Can you work these out from the model? Positions are in its coordinate system, mm. A direction names the side the tool comes from. Round coordinates to 2 decimals unless told otherwise and drop trailing zeros. Write each loop counter-clockwise with the first axis right and the second up, starting at its lowest first coordinate (ties: lowest second). Pieces come first, ordered by that corner, then holes. Notation, with made-up numbers: M 29,88 L 46,88 A9 ccw 46,103 Z; hole C 40,5.5 d7. An arc over 180 degrees is marked long. Answer as a JSON object with one key per item and string values. Group by question number.
1) Suppose I cut it at D-D, the plane y = -10. State how many separate pieces and enclosed holes the cut face has, and give its area (3 significant figures).
2) Suppose I cut it at B-B, the plane x = -49. Write out the boundary of the cut face in (y, z).
3) If we mould it in two halves opening along Y, with no side actions, what happens to faces 1 (the cylindrical face through (40.986, -6.025, 37.846)), 2 (the flat face through (41, -30.277, 49)), 3 (the flat face through (17, -4, 63))? For each: +Y half, -Y half, draft (parallel to the pull), parting line (faces both ways), or undercut.
4) On a 3-axis mill with a long thin cutter (end or side, diameter ignored), from which of +Z, -Z, +X, -X, +Y, -Y can I reach the whole of each face in a straight line? I mean faces 4 (the flat face through (-91, 2.723, 69)), 5 (the flat face through (-31, 6.873, 115)), 6 (the flat face through (-31, 5, 100)), 7 (the cylindrical face through (-39.773, -26.25, 0.74)). Say none if no direction works.
5) Please list where these lines run through material, in increasing order: L1, parallel to X at y = -25.5, z = 65; L2, parallel to X at y = -9, z = 114.5; L3, parallel to Y at x = -44, z = 41. Write a range as [from, to].
6) I'm going to push flat-ended pins straight in: pin 1 Ø12 at (x, z) = (0.5, 113.5) entering from -Y; pin 2 Ø1 at (x, z) = (-55, 109.5) entering from -Y; pin 3 Ø10 at (y, z) = (-8.5, 114.5) entering from -X. Where does each tip first touch, or does it pass through?
7) Suppose I cut it at C-C, the plane z = 45. Write out the boundary of the cut face in (x, y), and give its area (3 significant figures).
8) Suppose I cut it at A-A, the plane z = 106.5. Write out the boundary of the cut face in (x, y).
from build123d import *

# Parameters (mm, degrees)
BOSS_EXTRUDE2_DEPTH = 100
BOSS_EXTRUDE3_DEPTH = 30
SKETCH10_R          = 7.5
CUT_EXTRUDE2_DEPTH  = 210
SKETCH15_R          = 1.5
CUT_EXTRUDE3_DEPTH  = 10
SKETCH16_W          = 24
SKETCH16_H          = 12
BOSS_EXTRUDE5_DEPTH = 2
SKETCH17_W          = 3
SKETCH17_H          = 12
BOSS_EXTRUDE6_DEPTH = 25
SKETCH19_R          = 3.5
CUT_EXTRUDE4_DEPTH  = 1
SKETCH20_R          = 1.55
CUT_EXTRUDE5_DEPTH  = 3
SKETCH21_W          = 45
SKETCH21_H          = 1.5
BOSS_EXTRUDE7_DEPTH = 35
SKETCH23_R          = 8.25
CUT_EXTRUDE6_DEPTH  = 40
CUT_EXTRUDE7_DEPTH  = 40


with BuildPart() as part:
    # Sketch3 → Boss-Extrude2 (new body)
    with BuildSketch(Plane.XY):
        Polygon((-106.54853621, -30.277349769), (-106.54853621, 11.722650231), (43.45146379, 11.722650231), (43.45146379, -30.277349769), (38.45146379, -30.277349769), (38.45146379, 4.722650231), (-101.54853621, 4.722650231), (-101.54853621, -30.277349769), align=None)
    extrude(amount=BOSS_EXTRUDE2_DEPTH)

    # Sketch4 → Boss-Extrude3 (add)
    with BuildSketch(Plane.XY.offset(100)):
        with BuildLine():
            Line((-102.69853621, -0.277349769), (-102.69853621, -20.277349769))
            ThreePointArc((-102.69853621, -20.277349769), (-104.04853621, -21.627349769), (-105.39853621, -20.277349769))
            Line((-105.39853621, -20.277349769), (-105.39853621, -0.277349769))
            ThreePointArc((-105.39853621, -0.277349769), (-104.04853621, 1.072650231), (-102.69853621, -0.277349769))
        make_face()
        with BuildLine():
            Line((-56.54853621, 9.572650231), (-6.54853621, 9.572650231))
            ThreePointArc((-6.54853621, 9.572650231), (-5.19853621, 8.222650231), (-6.54853621, 6.872650231))
            Line((-6.54853621, 6.872650231), (-56.54853621, 6.872650231))
            ThreePointArc((-56.54853621, 6.872650231), (-57.89853621, 8.222650231), (-56.54853621, 9.572650231))
        make_face()
        with BuildLine():
            Line((42.45146379, -0.277349769), (42.45146379, -20.277349769))
            ThreePointArc((42.45146379, -20.277349769), (40.95146379, -21.777349769), (39.45146379, -20.277349769))
            Line((39.45146379, -20.277349769), (39.45146379, -0.277349769))
            ThreePointArc((39.45146379, -0.277349769), (40.95146379, 1.222650231), (42.45146379, -0.277349769))
        make_face()
    extrude(amount=BOSS_EXTRUDE3_DEPTH)

    # Sketch10 → Cut-Extrude2 (cut)
    with BuildSketch(Plane(origin=(43.45146379, 0, 0), x_dir=(0, 0, -1), z_dir=(1, 0, 0))):
        with Locations((-45, -8.277349769)):
            Circle(SKETCH10_R)
    extrude(amount=-CUT_EXTRUDE2_DEPTH, mode=Mode.SUBTRACT)

    # Sketch15 → Cut-Extrude3 (cut)
    with BuildSketch(Plane(origin=(0, 11.722650231, 0), x_dir=(1, 0, 0), z_dir=(0, 1, 0))):
        with Locations(Location((-31.54853621, -4.714245873, 0), (0, 0, 270))):
            Circle(SKETCH15_R)
    extrude(amount=-CUT_EXTRUDE3_DEPTH, mode=Mode.SUBTRACT)

    # Sketch16 → Boss-Extrude5 (add)
    with BuildSketch(Plane.XZ.offset(-4.722650231)):
        with Locations((26.45146379, 69)):
            Rectangle(SKETCH16_W, SKETCH16_H)
    boss_extrude5 = extrude(amount=BOSS_EXTRUDE5_DEPTH)

    # Sketch17 → Boss-Extrude6 (add)
    with BuildSketch(Plane(origin=(0, 2.722650231, 0), x_dir=(-1, 0, 0), z_dir=(0, -1, 0))):
        with Locations((-15.95146379, -69)):
            Rectangle(SKETCH17_W, SKETCH17_H)
    boss_extrude6 = extrude(amount=BOSS_EXTRUDE6_DEPTH)

    # Sketch19 → Cut-Extrude4 (cut)
    with BuildSketch(Plane.ZY.offset(-14.45146379)):
        with Locations((69.485133357, 0.222650231)):
            Circle(SKETCH19_R)
        with Locations((69.485133357, -17.777349769)):
            Circle(SKETCH19_R)
    cut_extrude4 = extrude(amount=-CUT_EXTRUDE4_DEPTH, mode=Mode.SUBTRACT)

    # Sketch20 → Cut-Extrude5 (cut)
    with BuildSketch(Plane.ZY.offset(-15.45146379)):
        with Locations((69.485133357, 0.222650231)):
            Circle(SKETCH20_R)
        with Locations((69.485133357, -17.777349769)):
            Circle(SKETCH20_R)
    cut_extrude5 = extrude(amount=-CUT_EXTRUDE5_DEPTH, mode=Mode.SUBTRACT)

    # Mirror6: Boss-Extrude5, Boss-Extrude6, Cut-Extrude4, Cut-Extrude5 across plane
    add(boss_extrude5.mirror(Plane.ZY.offset(31.54853621)))
    add(boss_extrude6.mirror(Plane.ZY.offset(31.54853621)))
    add(cut_extrude4.mirror(Plane.ZY.offset(31.54853621)), mode=Mode.SUBTRACT)
    add(cut_extrude5.mirror(Plane.ZY.offset(31.54853621)), mode=Mode.SUBTRACT)

    # Sketch21 → Boss-Extrude7 (add)
    with BuildSketch(Plane.XZ.offset(-4.722650231)):
        with Locations((-31.54853621, 0.75)):
            Rectangle(SKETCH21_W, SKETCH21_H)
    extrude(amount=BOSS_EXTRUDE7_DEPTH)

    # Sketch23 → Cut-Extrude6 (cut)
    with BuildSketch(Plane(origin=(0, 0, 0), x_dir=(-1, 0, 0), z_dir=(0, 0, -1))):
        with Locations((44.54853621, -16.277349769)):
            Circle(SKETCH23_R)
        with Locations((18.54853621, -16.277349769)):
            Circle(SKETCH23_R)
    extrude(amount=-CUT_EXTRUDE6_DEPTH, mode=Mode.SUBTRACT)

    # Sketch24 → Cut-Extrude7 (cut)
    with BuildSketch(Plane(origin=(0, 0, 0), x_dir=(-1, 0, 0), z_dir=(0, 0, -1))):
        with BuildLine():
            Line((26.54853621, -23.095326639), (36.54853621, -23.095326639))
            ThreePointArc((36.54853621, -23.095326639), (39.773941895, -26.320732325), (36.54853621, -29.54613801))
            Line((36.54853621, -29.54613801), (26.54853621, -29.54613801))
            ThreePointArc((26.54853621, -29.54613801), (23.323130524, -26.320732325), (26.54853621, -23.095326639))
        make_face()
    extrude(amount=-CUT_EXTRUDE7_DEPTH, mode=Mode.SUBTRACT)


solid = part.part
Results:
{
 "1": {"separate pieces": "9", "enclosed holes": "0", "area": "1,130 mm^2"},
 "2": {"outline": "M -30.28,0 L -23.22,0 L -23.22,1.5 L -30.28,1.5 Z; M -9.33,0 L 11.72,0 L 11.72,100 L 9.57,100 L 9.57,130 L 6.87,130 L 6.87,100 L 4.72,100 L 4.72,1.5 L -9.33,1.5 Z"},
 "3": {"face 1": "undercut", "face 2": "-Y half", "face 3": "draft"},
 "4": {"face 4": "+Z, -Z, -Y", "face 5": "+Z, +X, -X, -Y", "face 6": "+Z", "face 7": "+Z, -Z"},
 "5": {"L1": "[-106.55, -101.55], [38.45, 43.45]", "L2": "[-105.4, -102.7], [39.45, 42.45]", "L3": "[4.72, 11.72]"},
 "6": {"pin 1": "y = 7.37", "pin 2": "y = 6.87", "pin 3": "x = -105.4"},
 "7": {"outline": "M -106.55,-30.28 L -101.55,-30.28 L -101.55,-15.78 L -106.55,-15.78 Z; M -106.55,-0.78 L -101.55,-0.78 L -101.55,4.72 L 38.45,4.72 L 38.45,-0.78 L 43.45,-0.78 L 43.45,11.72 L -106.55,11.72 Z; M 38.45,-30.28 L 43.45,-30.28 L 43.45,-15.78 L 38.45,-15.78 Z", "area": "1,250 mm^2"},
 "8": {"outline": "M -105.4,-20.28 A1.35 ccw -102.7,-20.28 L -102.7,-0.28 A1.35 ccw -105.4,-0.28 Z; M -56.55,6.87 L -6.55,6.87 A1.35 ccw -6.55,9.57 L -56.55,9.57 A1.35 ccw Z; M 39.45,-20.28 A1.5 ccw 42.45,-20.28 L 42.45,-0.28 A1.5 ccw 39.45,-0.28 Z"}
}
